The model under review builds one solid part; all positions refer to its coordinate system, in mm. A direction names the side the tool comes from. Coordinates: 2 decimals unless noted, no trailing zeros. Write each loop counter-clockwise with the first axis right and the second up, starting at its lowest first coordinate (ties: lowest second). Pieces come first, ordered by that corner, then holes.
```python
from build123d import *

# Parameters (mm, degrees)
SKIZZE1_R                       = 11.5
AUFSATZ_LINEAR_AUSTRAGEN1_DEPTH = 77
SCHNITT_LINEAR_AUSTRAGEN1_DEPTH = 4.1
SKIZZE3_R                       = 2.1
SCHNITT_LINEAR_AUSTRAGEN2_DEPTH = 3
SKIZZE4_R                       = 9.6
SCHNITT_LINEAR_AUSTRAGEN3_DEPTH = 12.75
SCHNITT_LINEAR_START            = -6
SKIZZE7_W                       = 1.5
SKIZZE7_H                       = 15
SCHNITT_LINEAR_AUSTRAGEN4_DEPTH = 63
SKIZZE8_W                       = 63
SKIZZE8_H                       = 4
AUFSATZ_LINEAR_AUSTRAGEN2_DEPTH = 1.5
SCHNITT_LINEAR_AUSTRAGEN6_DEPTH = 13.5
SKIZZE12_R                      = 3
SCHNITT_LINEAR_AUSTRAGEN7_DEPTH = 2
KREISMUSTER3_COUNT              = 3
SKIZZE13_R                      = 8.5
SCHNITT_LINEAR_AUSTRAGEN8_DEPTH = 40


with BuildPart() as part:
    # Skizze1 → Aufsatz-Linear austragen1 (new body)
    with BuildSketch(Plane(origin=(0, 0, 0), x_dir=(0, 0, -1), z_dir=(1, 0, 0))):
        Circle(SKIZZE1_R)
    extrude(amount=AUFSATZ_LINEAR_AUSTRAGEN1_DEPTH)

    # Skizze2 → Schnitt-Linear austragen1 (cut)
    with BuildSketch(Plane(origin=(77, 0, 0), x_dir=(0, 0, -1), z_dir=(1, 0, 0))):
        with BuildLine():
            Line((-6.942668977, 1.486387391), (-6.842668977, 1.486387391))
            Line((-6.842668977, 1.486387391), (-6.842668977, -1.513612609))
            Line((-6.842668977, -1.513612609), (-6.936784332, -1.513612609))
            ThreePointArc((-6.936784332, -1.513612609), (-5.735823545, -4.184534414), (-3.559041115, -6.143551607))
            Line((-3.559041115, -6.143551607), (-3.528139415, -6.048445955))
            Line((-3.528139415, -6.048445955), (-0.674969866, -6.975496938))
            Line((-0.674969866, -6.975496938), (-0.70405311, -7.06500596))
            ThreePointArc((-0.70405311, -7.06500596), (2.207261771, -6.748184606), (4.743060601, -5.283311096))
            Line((4.743060601, -5.283311096), (4.662158901, -5.224532571))
            Line((4.662158901, -5.224532571), (6.425514658, -2.797481588))
            Line((6.425514658, -2.797481588), (6.50165558, -2.852801206))
            ThreePointArc((6.50165558, -2.852801206), (7.099986341, 0.013926966), (6.490413777, 2.878285776))
            Line((6.490413777, 2.878285776), (6.409512077, 2.819507251))
            Line((6.409512077, 2.819507251), (4.64615632, 5.246558234))
            Line((4.64615632, 5.246558234), (4.722297242, 5.301877852))
            ThreePointArc((4.722297242, 5.301877852), (2.180771108, 6.756791944), (-0.731764286, 7.062189535))
            Line((-0.731764286, 7.062189535), (-0.700862586, 6.967083883))
            Line((-0.700862586, 6.967083883), (-3.554032135, 6.0400329))
            Line((-3.554032135, 6.0400329), (-3.583115379, 6.129541922))
            ThreePointArc((-3.583115379, 6.129541922), (-5.752195675, 4.162000111), (-6.942668977, 1.486387391))
        make_face()
    extrude(amount=-SCHNITT_LINEAR_AUSTRAGEN1_DEPTH, mode=Mode.SUBTRACT)

    # Skizze3 → Schnitt-Linear austragen2 (cut)
    with BuildSketch(Plane(origin=(72.9, 0, 0), x_dir=(0, 0, -1), z_dir=(1, 0, 0))):
        Circle(SKIZZE3_R)
    extrude(amount=-SCHNITT_LINEAR_AUSTRAGEN2_DEPTH, mode=Mode.SUBTRACT)

    # Skizze4 → Schnitt-Linear austragen3 (cut)
    with BuildSketch(Plane.ZY):
        Circle(SKIZZE4_R)
    extrude(amount=-SCHNITT_LINEAR_AUSTRAGEN3_DEPTH, mode=Mode.SUBTRACT)

    # Skizze7 → Schnitt-Linear austragen4 (cut)
    with BuildSketch(Plane(origin=(77, 0, 0), x_dir=(0, 0, -1), z_dir=(1, 0, 0)).offset(SCHNITT_LINEAR_START)):
        with Locations((-10.75, 0)):
            Rectangle(SKIZZE7_W, SKIZZE7_H)
    schnitt_linear_austragen4 = extrude(amount=-SCHNITT_LINEAR_AUSTRAGEN4_DEPTH, mode=Mode.SUBTRACT)

    # Skizze8 → Aufsatz-Linear austragen2 (add)
    with BuildSketch(Plane.XY.offset(10)):
        with Locations((39.5, 0)):
            Rectangle(SKIZZE8_W, SKIZZE8_H)
    aufsatz_linear_austragen2 = extrude(amount=AUFSATZ_LINEAR_AUSTRAGEN2_DEPTH)

    # Skizze10 → Schnitt-Linear austragen6 (cut)
    with BuildSketch(Plane.ZY.offset(-12.75)):
        Polygon((4.038863706, -2.240739453), (3.959969143, 2.377388845), (-0.078894563, 4.618128298), (-4.038863706, 2.240739453), (-3.959969143, -2.377388845), (0.078894563, -4.618128298), align=None)
    extrude(amount=-SCHNITT_LINEAR_AUSTRAGEN6_DEPTH, mode=Mode.SUBTRACT)

    # Skizze12 → Schnitt-Linear austragen7 (cut)
    with BuildSketch(Plane.ZY.offset(-26.25)):
        Circle(SKIZZE12_R)
    extrude(amount=-SCHNITT_LINEAR_AUSTRAGEN7_DEPTH, mode=Mode.SUBTRACT)

    # Kreismuster3: Schnitt-Linear austragen4, Aufsatz-Linear austragen2 ×3 about axis
    kreismuster3_axis = Axis((0, 0, 0), (1, 0, 0))
    add([schnitt_linear_austragen4.rotate(kreismuster3_axis, i * 360 / KREISMUSTER3_COUNT) for i in range(1, KREISMUSTER3_COUNT)], mode=Mode.SUBTRACT)
    add([aufsatz_linear_austragen2.rotate(kreismuster3_axis, i * 360 / KREISMUSTER3_COUNT) for i in range(1, KREISMUSTER3_COUNT)])

    # Skizze13 → Schnitt-Linear austragen8 (cut)
    with BuildSketch(Plane(origin=(69.9, 0, 0), x_dir=(0, 0, -1), z_dir=(1, 0, 0))):
        Circle(SKIZZE13_R)
    extrude(amount=-SCHNITT_LINEAR_AUSTRAGEN8_DEPTH, mode=Mode.SUBTRACT)


solid = part.part
```
Item 1: Take a section at A-A, the plane x = 56.5. Write out the cut boundary in (y, z), plus the area to 3 significant figures.
Solved:
outline: (-11.5, -0.08) - (-9.66, -3.27) - (-10.96, -4.02) - (-8.96, -7.48) - (-7.66, -6.73) - (-5.82, -9.92) arc R11.5 ccw to (5.82, -9.92) - (7.66, -6.73) - (8.96, -7.48) - (10.96, -4.02) - (9.66, -3.27) - (11.5, -0.08) arc R11.5 ccw to (5.68, 10) - (2, 10) - (2, 11.5) - (-2, 11.5) - (-2, 10) - (-5.68, 10) arc R11.5 ccw to start; hole circle Ø17 at (0, 0)
area: 172 mm2
Item 2: Mouldability with a two-part tool opening along Z and no side actions: class faces 1 (the face through (75, 0, 6.843)), 2 (the face through (38, 11.4, 1.5)), 3 (the face through (71, -3.4, 10.5)), 4 (the face through (39.941, -6.728, -8.347)) as pulls with the +Z half, pulls with the -Z half, needs draft (parallel to the pull), parting line crosses it, or undercut.
Solved:
face 1: undercut
face 2: parting line crosses it
face 3: needs draft
face 4: pulls with the -Z half
Item 3: Take a section at C-C, the plane x = 72. Write out the cut boundary in (y, z).
Solved:
outline: circle Ø23 at (0, 0); hole circle Ø4.2 at (0, 0)
Item 4: To check wall thickness, follow line 1 along Y through (x, z) = (6, -7.75); line 2 along X through (y, z) = (1, 3.75); line 3 along X through (y, z) = (4.5, 6.25). State the ranges of each line that lie inside material, in increasing order.
Solved:
line 1: y = -8.5 to -5.67, 5.67 to 8.5
line 2: x = 26.25 to 29.9, 69.9 to 72.9
line 3: x = 12.75 to 29.9, 69.9 to 77
Item 5: For pin 1 (1.5 mm diameter, centred on x = 68, y = 3, fed in from +Z); pin 2 (1.5 mm diameter, centred on x = 63.5, y = -7, fed in from +Z); pin 3 (1.5 mm diameter, centred on y = 1.5, z = -7.5, fed in from -X), all flat-tipped, find the tip position at first contact; note any pin that passes through.
Solved:
pin 1: stops at z = 10
pin 2: stops at z = 9.65
pin 3: stops at x = 12.75
Item 6: Take a section at B-B, the plane x = 25. Write out the cut boundary in (y, z), plus the area to 3 significant figures.
Solved:
outline: (-11.5, -0.08) - (-9.66, -3.27) - (-10.96, -4.02) - (-8.96, -7.48) - (-7.66, -6.73) - (-5.82, -9.92) arc R11.5 ccw to (5.82, -9.92) - (7.66, -6.73) - (8.96, -7.48) - (10.96, -4.02) - (9.66, -3.27) - (11.5, -0.08) arc R11.5 ccw to (5.68, 10) - (2, 10) - (2, 11.5) - (-2, 11.5) - (-2, 10) - (-5.68, 10) arc R11.5 ccw to start; hole (-4.62, 0.08) - (-2.38, -3.96) - (2.24, -4.04) - (4.62, -0.08) - (2.38, 3.96) - (-2.24, 4.04) - close
area: 344 mm2
Item 7: Machinability: for faces 5 (the face through (8, 7.4, -8.3)), 6 (the face through (74.98, 6.51, 2.11)), 7 (the face through (29.9, 0, 0)), 8 (the face through (19.41, 3.48, 1.97)), 9 (the face through (8, -11, -2)), which of the approach directions +Z, -Z, +X, -X, +Y, -Y give a long, thin tool a straight path to every point of the face, cutting with its end or side? Answer none if there is none.
Solved:
face 5: -Z
face 6: +X
face 7: none
face 8: -X
face 9: -Y
